Check sheet for the modelled part. Datum: model origin and axes. Units: mm. Face numbers are marked on the shaded views. A direction names the side the tool comes from. Give positions to 0.01 mm unless a question says otherwise; leave off trailing zeros. Order: outer loops, then holes, each group sorted by start corner. A loop starts at its lowest first (then second) coordinate and runs counter-clockwise, first axis right, second up. Notation, with made-up numbers: M 73,-26 L 128,-26 A16 cw 128,-3 Z; hole C 24.25,-1.5 d6. An arc over 180 degrees is marked long. One line per question, with ' | ' between items. Start each with the question number.
```python
from build123d import *

# Parameters (mm, degrees)
F0_W     = 914.4
F0_H     = 609.6
F0_W_2   = 863.6
F0_H_2   = 558.8
F1_DEPTH = 127
F2_R     = 177.8
F3_DEPTH = 38.1


with BuildPart() as f1:
    # F0 (on Top) → F1 (new body)
    with BuildSketch(Plane.XY):
        Rectangle(F0_W, F0_H)
        Rectangle(F0_W_2, F0_H_2, mode=Mode.SUBTRACT)
    extrude(amount=F1_DEPTH)

    # F2 (on face) → F3 (join)
    with BuildSketch(Plane.XZ.offset(-279.4)):
        with Locations((-241.3, 50.8)):
            Circle(F2_R)
        with Locations((241.3, 50.8)):
            Circle(F2_R)
    extrude(amount=F3_DEPTH)

    # F4: F1 across plane


with BuildPart() as f1_1:
    add(f1.part)
    add(f1.part.mirror(Plane.XZ))


solid = f1_1.part
```
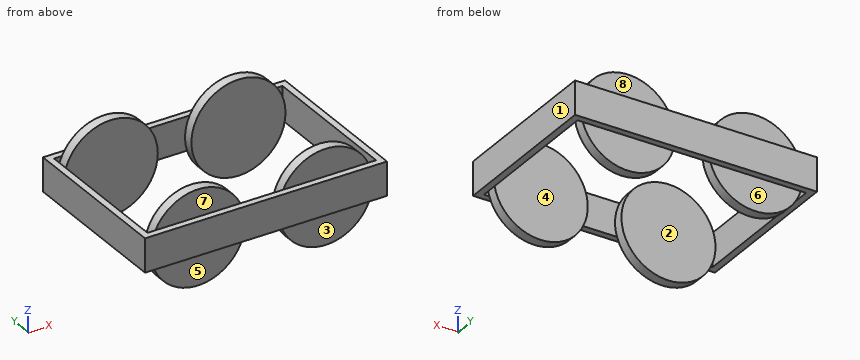
Item 1: Section check D-D, the plane x = -34. Record the cut outline in (y, z).
Item 2: Section check B-B, the plane y = 95. Record the cut outline in (x, z), then the cut area to 3 significant figures.
Item 3: Draft check along Y on the marked faces 1, 2 and 3. Enter one of: released by +Y, released by -Y, zero draft, split by the parting line, or undercut.
Item 4: Section check C-C, the plane z = 50.8. Record the cut outline in (x, y).
Item 5: Scan lines: probe 1 along Y at (x, z) = (-287.5, -34.5); probe 2 along Y at (x, z) = (55.5, 20.5); probe 3 along X at (y, z) = (-248, 30.5). Record each from-to range of solid material in increasing order. Write a range as [from, to].
Item 6: Section check A-A, the plane x = -241.3. Record the cut outline in (y, z).
Item 7: Go/stop test with a flat-tipped pin: P1, Ø8, axis at x = 217.5, z = -36, coming from the -Y side. Record where the tip stops, or that it passes through.
Item 8: Set-up check for the marked faces 4, 5, 6, 7 and 8: record each of +Z, -Z, +X, -X, +Y, -Y from which the full face is reachable in a straight line by a thin tool's end or side.
Reported:
1) outline: M -304.8,0 L -279.4,0 L -279.4,127 L -304.8,127 Z; M 279.4,0 L 304.8,0 L 304.8,127 L 279.4,127 Z
2) outline: M -457.2,0 L -431.8,0 L -431.8,127 L -457.2,127 Z; M 431.8,0 L 457.2,0 L 457.2,127 L 431.8,127 Z | area: 6,450 mm^2
3) face 1: zero draft | face 2: undercut | face 3: released by -Y
4) outline: M -457.2,-304.8 L 457.2,-304.8 L 457.2,304.8 L -457.2,304.8 Z; hole M -431.8,-279.4 L -419.1,-279.4 L -419.1,-241.3 L -63.5,-241.3 L -63.5,-279.4 L 63.5,-279.4 L 63.5,-241.3 L 419.1,-241.3 L 419.1,-279.4 L 431.8,-279.4 L 431.8,279.4 L 419.1,279.4 L 419.1,241.3 L 63.5,241.3 L 63.5,279.4 L -63.5,279.4 L -63.5,241.3 L -419.1,241.3 L -419.1,279.4 L -431.8,279.4 Z
5) probe 1: y = [-279.4, -241.3], [241.3, 279.4] | probe 2: y = [-304.8, -279.4], [279.4, 304.8] | probe 3: x = [-457.2, -431.8], [-417.94, -64.66], [64.66, 417.94], [431.8, 457.2]
6) outline: M -304.8,0 L -279.4,0 L -279.4,-127 L -241.3,-127 L -241.3,228.6 L -279.4,228.6 L -279.4,127 L -304.8,127 Z; M 241.3,-127 L 279.4,-127 L 279.4,0 L 304.8,0 L 304.8,127 L 279.4,127 L 279.4,228.6 L 241.3,228.6 Z
7) P1: stops at y = -279.4
8) face 4: +Z, -Z | face 5: -Z, +X, -X, -Y | face 6: -Z, +X, -X, +Y | face 7: +Z, +X, -X, -Y | face 8: +Z, +X, -X, +Y
